Answer from the drawing. Dimensions are ordinates in mm from the lowest x, y and z of the part. A direction names the side the tool comes from. Coordinates: 2 decimals unless noted, no trailing zeros. Write each loop counter-clockwise with the first axis right and the second up, starting at its lowest first coordinate (ties: lowest second). Pieces come first, ordered by that corner, then holes.
(1) The part is cut by section A-A, the plane x = 47.5. Determine the outline of the cut face in (y, z) (1 decimal), and give its area (3 significant figures).
(2) Given pin 1 (8 mm diameter, centred on x = 49, y = 85, fed in from -Z); pin 2 (5 mm diameter, centred on y = 32.5, z = 80.5, fed in from +X); pin 3 (10 mm diameter, centred on x = 83, y = 76.5, fed in from -Z), each flat-ended and moving along its own axis, determine where each tip first touches the part or whether it passes through.
(3) The part is cut by section C-C, the plane y = 52.5. Determine the outline of the cut face in (x, z) (1 decimal).
(4) Straight lines are drawn through the part: line 1 along Y through (x, z) = (54, 26.5); line 2 along Y through (x, z) = (57, 11) (1 decimal); line 3 along X through (y, z) = (60.5, 101.5) (1 decimal). For each, find the intervals that lie inside material, in ascending order.
(5) Which of the six approach directions +Z, -Z, +X, -X, +Y, -Y give full straight-line access (tool end or side, diameter ignored) to the marked faces 1 and 2?
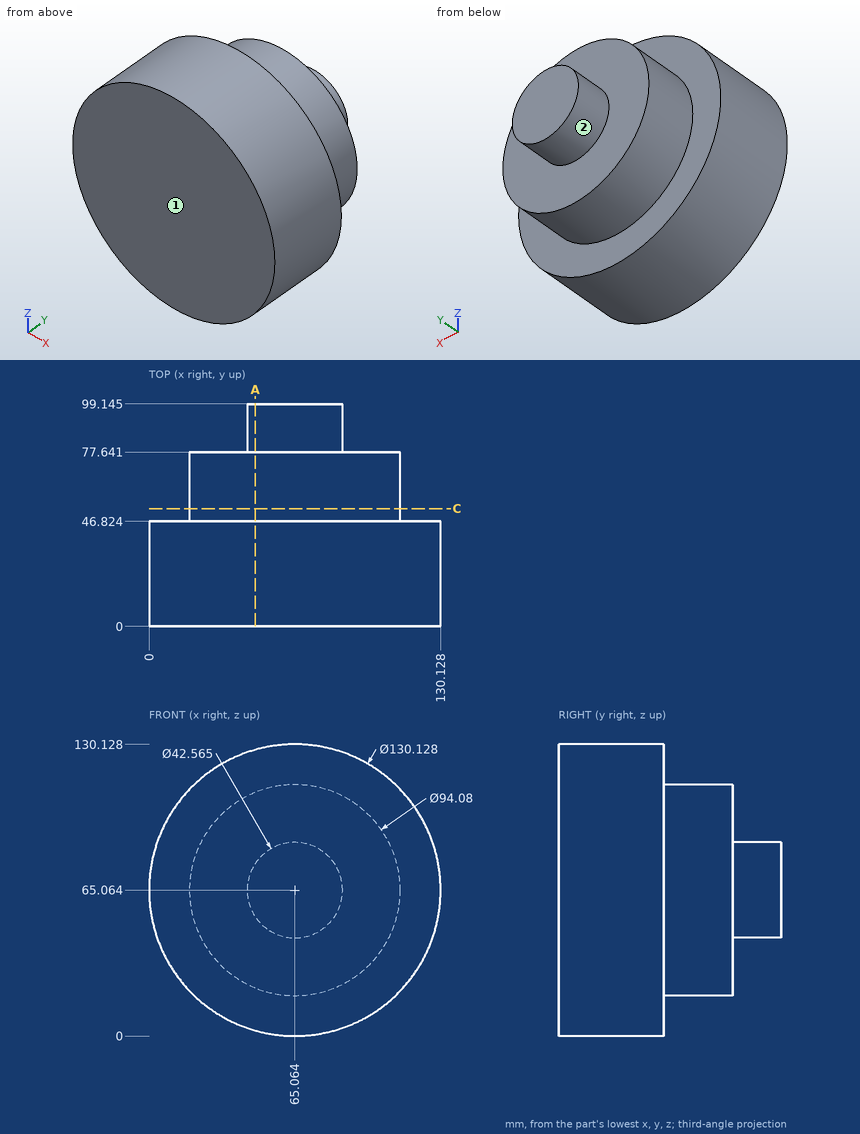
Computed:
1. outline: (0, 2.4) - (46.8, 2.4) - (46.8, 21.4) - (77.6, 21.4) - (77.6, 53) - (99.1, 53) - (99.1, 77.1) - (77.6, 77.1) - (77.6, 108.7) - (46.8, 108.7) - (46.8, 127.7) - (0, 127.7) - close
1. area: 9,070 mm2
2. pin 1: stops at z = 47.53
2. pin 2: stops at x = 128.83
2. pin 3: stops at z = 19.84
3. outline: circle Ø94.1 at (65.1, 65.1)
4. line 1: y = 0 to 77.64
4. line 2: y = 0 to 46.8
4. line 3: x = 35.3 to 94.8
5. face 1: +Z, -Z, +X, -X, -Y
5. face 2: +Y
